```python
from build123d import *

# Parameters (mm, degrees)
ESBO_O1_R                = 7
ESBO_O1_W                = 100
ESBO_O1_H                = 14
RESSALTO_EXTRUS_O1_DEPTH = 20
ESBO_O2_R                = 4
CORTE_EXTRUS_O1_DEPTH    = 20
ESBO_O3_W                = 10
ESBO_O3_H                = 2
CORTE_EXTRUS_O2_DEPTH    = 20
ESBO_O4_W                = 8
ESBO_O4_H                = 3
RESSALTO_EXTRUS_O2_DEPTH = 20
ESBO_O5_R                = 1.5
CORTE_EXTRUS_O3_DEPTH    = 20


with BuildPart() as part:
    # Esboço1 → Ressalto-extrusão1 (new body)
    with BuildSketch(Plane(origin=(0, 0, 0), x_dir=(1, 0, 0), z_dir=(0, 1, 0))):
        with Locations((0, 7)):
            Circle(ESBO_O1_R)
        with Locations((50, 7)):
            Rectangle(ESBO_O1_W, ESBO_O1_H)
    extrude(amount=RESSALTO_EXTRUS_O1_DEPTH)

    # Esboço2 → Corte-extrusão1 (cut)
    with BuildSketch(Plane(origin=(0, 20, 0), x_dir=(1, 0, 0), z_dir=(0, 1, 0))):
        with Locations(Location((0, 7, 0), (0, 0, 270))):
            Circle(ESBO_O2_R)
    extrude(amount=-CORTE_EXTRUS_O1_DEPTH, mode=Mode.SUBTRACT)

    # Esboço3 → Corte-extrusão2 (cut)
    with BuildSketch(Plane(origin=(0, 20, 0), x_dir=(1, 0, 0), z_dir=(0, 1, 0))):
        with Locations((-4, 7)):
            Rectangle(ESBO_O3_W, ESBO_O3_H)
    extrude(amount=-CORTE_EXTRUS_O2_DEPTH, mode=Mode.SUBTRACT)

    # Esboço4 → Ressalto-extrusão2 (add)
    with BuildSketch(Plane(origin=(0, 20, 0), x_dir=(1, 0, 0), z_dir=(0, 1, 0))):
        with Locations((-7.872983346, 9.5)):
            Rectangle(ESBO_O4_W, ESBO_O4_H)
        with Locations((-7.872983346, 4.5)):
            Rectangle(ESBO_O4_W, ESBO_O4_H)
    extrude(amount=-RESSALTO_EXTRUS_O2_DEPTH)

    # Esboço5 → Corte-extrusão3 (cut)
    with BuildSketch(Plane.XY.offset(-3)):
        with Locations((-8.872983346, 15)):
            Circle(ESBO_O5_R)
        with Locations((-8.872983346, 5)):
            Circle(ESBO_O5_R)
    extrude(amount=-CORTE_EXTRUS_O3_DEPTH, mode=Mode.SUBTRACT)


solid = part.part
```
Can you work these out from the model? Positions are in its coordinate system, mm. A direction names the side the tool comes from. Give positions to 0.01 mm unless a question says otherwise; leave off trailing zeros. Loops run counter-clockwise (first coordinate to the right, second up) from the corner with the lowest first, then second, coordinate; pieces in that order, holes last. Notation, with made-up numbers: M 38.5,49.25 L 49.5,49.25 A22 ccw 49.5,70.25 Z; hole C -10,38 d10. An arc over 180 degrees is marked long. One line per item, written item: value.
(1) Suppose I cut it at A-A on y = 15. List the corners of the cut face in (x, z) for me, plus the area to 3 significant figures.
Returned:
outline: M -11.87,-11 L -10.37,-11 L -10.37,-8 L -11.87,-8 Z; M -11.87,-6 L -10.37,-6 L -10.37,-3 L -11.87,-3 Z; M -7.37,-11 L -5.74,-11 A7 ccw 0,-14 L 100,-14 L 100,0 L 0,0 A7 ccw -5.74,-3 L -7.37,-3 L -7.37,-6 L -3.87,-6 A4 cw long -3.87,-8 L -7.37,-8 Z
area: 1,440 mm^2
(2) Will these pins go through, and if not, where does the flat tip stop? pin 1 (4 mm diameter, centred on x = 1.5, z = -10, fed in from +Y); pin 2 (9 mm diameter, centred on x = -9, y = 9, fed in from +Z); pin 3 (4 mm diameter, centred on x = -8.87, y = 5, fed in from -Z); pin 4 (1.8 mm diameter, centred on x = -9.5, y = 8, fed in from +Z).
Returned:
pin 1: y = 20
pin 2: z = -1.64
pin 3: z = -11
pin 4: z = -3
(3) Which directions (+Z, -Z, +X, -X, +Y, -Y) give clear straight access to the entire face, cutting with the end or side of a thin tool? Please do faces 1 (the face through (-9, 10, -11)), 2 (the face through (-8, 10, -6)), 3 (the face through (-11.873, 10, -9)).
Returned:
face 1: -Z, -X, +Y, -Y
face 2: -X, +Y, -Y
face 3: +Z, -Z, -X, +Y, -Y
(4) Suppose I cut it at C-C on z = -9.75. List the corners of the cut face in (x, y) for me.
Returned:
outline: M -11.87,0 L -2.9,0 L -2.9,20 L -11.87,20 Z; M 2.9,0 L 100,0 L 100,20 L 2.9,20 Z; hole C -8.87,5 d3; hole C -8.87,15 d3
(5) Suppose I cut it at B-B on z = -4.75. List the corners of the cut face in (x, y) for me.
Returned:
outline: M -11.87,0 L -3.31,0 L -3.31,20 L -11.87,20 Z; M 3.31,0 L 100,0 L 100,20 L 3.31,20 Z; hole C -8.87,5 d3; hole C -8.87,15 d3
(6) I need wall thicknesses on line 1 (Z direction, x = -7, y = 13); line 2 (X direction, y = 14.5, z = -7); line 3 (Z direction, x = 0, y = 14.25). Which ranges of each line are inside material? Lowest first, please.
Returned:
line 1: -11 to -8, -6 to -3
line 2: 4 to 100
line 3: -14 to -11, -3 to 0
(7) We'd pull the mould along X, two halves only. Please class faces 4 (the face through (100, 10, -7)), 5 (the face through (-3.282, 9.86, -0.817)), 6 (the face through (-7.5, 14.4, -9.5)), 7 (the face through (-9, 10, -3)): released by +X, released by -X, zero draft, split by the parting line, or undercut.
Returned:
face 4: released by +X
face 5: released by -X
face 6: undercut
face 7: zero draft
